```python
from build123d import *

# Parameters (mm, degrees)
SKETCH1_W           = 116.070000016
SKETCH1_H           = 84.320000016
BOSS_EXTRUDE1_DEPTH = 2.54
SKETCH2_W           = 116.070000016
SKETCH2_H           = 84.320000016
SKETCH2_W_2         = 108.450000016
SKETCH2_H_2         = 76.700000016
BOSS_EXTRUDE2_DEPTH = 34.925
CUT_EXTRUDE1_START  = 0.25
SKETCH4_R           = 1.349999967
CUT_EXTRUDE1_DEPTH  = 3.81
CUT_EXTRUDE2_START  = 0.25
SKETCH5_R           = 1.349999967
CUT_EXTRUDE2_DEPTH  = 3.81
SKETCH7_R           = 2.999999969
CUT_EXTRUDE3_DEPTH  = 2.000000064
SKETCH6_R           = 2.999999969
CUT_EXTRUDE4_DEPTH  = 2.000000064
CUT_EXTRUDE5_START  = 0.25
SKETCH11_W          = 22.225
SKETCH11_H          = 22.86
CUT_EXTRUDE5_DEPTH  = 3.81
CUT_EXTRUDE6_START  = 0.25
SKETCH8_W           = 22.225
SKETCH8_H           = 25.4
CUT_EXTRUDE6_DEPTH  = 3.81
CUT_EXTRUDE7_START  = 0.25
SKETCH10_W          = 22.225
SKETCH10_H          = 22.86
CUT_EXTRUDE7_DEPTH  = 3.81


with BuildPart() as part:
    # Sketch1 → Boss-Extrude1 (new body)
    with BuildSketch(Plane.YZ):
        Rectangle(SKETCH1_W, SKETCH1_H)
    extrude(amount=BOSS_EXTRUDE1_DEPTH)

    # Sketch2 → Boss-Extrude2 (add)
    with BuildSketch(Plane(origin=(0, 0, 0), x_dir=(0, -1, 0), z_dir=(-1, 0, 0))):
        Rectangle(SKETCH2_W, SKETCH2_H)
        Rectangle(SKETCH2_W_2, SKETCH2_H_2, mode=Mode.SUBTRACT)
    extrude(amount=BOSS_EXTRUDE2_DEPTH)

    # Sketch4 → Cut-Extrude1 (cut)
    with BuildSketch(Plane.XZ.offset(53.975).offset(CUT_EXTRUDE1_START)):
        with Locations((-28.575, 31.75)):
            Circle(SKETCH4_R)
        with Locations((-28.575, -31.75)):
            Circle(SKETCH4_R)
    extrude(amount=CUT_EXTRUDE1_DEPTH, mode=Mode.SUBTRACT)

    # Sketch5 → Cut-Extrude2 (cut)
    with BuildSketch(Plane(origin=(0, 53.975, 0), x_dir=(-1, 0, 0), z_dir=(0, 1, 0)).offset(CUT_EXTRUDE2_START)):
        with Locations((28.575, -31.75)):
            Circle(SKETCH5_R)
        with Locations((28.575, 31.75)):
            Circle(SKETCH5_R)
    extrude(amount=CUT_EXTRUDE2_DEPTH, mode=Mode.SUBTRACT)

    # Sketch7 → Cut-Extrude3 (cut)
    with BuildSketch(Plane(origin=(0, 58.035000008, 0), x_dir=(-1, 0, 0), z_dir=(0, 1, 0))):
        with Locations((28.575, -31.75)):
            Circle(SKETCH7_R)
        with Locations((28.575, 31.75)):
            Circle(SKETCH7_R)
    extrude(amount=-CUT_EXTRUDE3_DEPTH, mode=Mode.SUBTRACT)

    # Sketch6 → Cut-Extrude4 (cut)
    with BuildSketch(Plane.XZ.offset(58.035000008)):
        with Locations((-28.575, 31.75)):
            Circle(SKETCH6_R)
        with Locations((-28.575, -31.75)):
            Circle(SKETCH6_R)
    extrude(amount=-CUT_EXTRUDE4_DEPTH, mode=Mode.SUBTRACT)

    # Sketch11 → Cut-Extrude5 (cut)
    with BuildSketch(Plane(origin=(0, 0, -38.1), x_dir=(1, 0, 0), z_dir=(0, 0, -1)).offset(CUT_EXTRUDE5_START)):
        with Locations((-11.1125, 34.925)):
            Rectangle(SKETCH11_W, SKETCH11_H)
    extrude(amount=CUT_EXTRUDE5_DEPTH, mode=Mode.SUBTRACT)

    # Sketch8 → Cut-Extrude6 (cut)
    with BuildSketch(Plane.XZ.offset(53.975).offset(CUT_EXTRUDE6_START)):
        with Locations((-11.1125, -12.7)):
            Rectangle(SKETCH8_W, SKETCH8_H)
    extrude(amount=CUT_EXTRUDE6_DEPTH, mode=Mode.SUBTRACT)

    # Sketch10 → Cut-Extrude7 (cut)
    with BuildSketch(Plane.XY.offset(38.1).offset(CUT_EXTRUDE7_START)):
        with Locations((-11.1125, -34.925)):
            Rectangle(SKETCH10_W, SKETCH10_H)
    extrude(amount=CUT_EXTRUDE7_DEPTH, mode=Mode.SUBTRACT)


solid = part.part
```
Geometry check sheet. Reference: the model listing, model coordinates, mm. A direction names the side the tool comes from. Round coordinates to 2 decimals unless told otherwise and drop trailing zeros. Order: outer loops, then holes, each group sorted by start corner. A loop starts at its lowest first (then second) coordinate and runs counter-clockwise, first axis right, second up. Notation, with made-up numbers: M -26.75,-10.5 L 23.25,-10.5 A15 ccw 23.25,-2.5 Z; hole C 59,32.25 d5. An arc over 180 degrees is marked long. Answer as CSV lines item,"result".
1) Sectioned sample at C-C on z = 31.75. Record the cut outline in (x, y) (3 decimals).
Entries:
outline,"M -34.925,-58.035 L -31.575,-58.035 L -31.575,-56.035 L -29.925,-56.035 L -29.925,-54.225 L -34.925,-54.225 Z; M -34.925,54.225 L -29.925,54.225 L -29.925,56.035 L -31.575,56.035 L -31.575,58.035 L -34.925,58.035 Z; M -27.225,-56.035 L -25.575,-56.035 L -25.575,-58.035 L 2.54,-58.035 L 2.54,58.035 L -25.575,58.035 L -25.575,56.035 L -27.225,56.035 L -27.225,54.225 L 0,54.225 L 0,-54.225 L -27.225,-54.225 Z"
2) Sectioned sample at A-A on z = -18. Record the cut outline in (x, y) (3 decimals), and give its area (3 significant figures).
Entries:
outline,"M -34.925,-58.035 L -22.225,-58.035 L -22.225,-54.225 L -34.925,-54.225 Z; M -34.925,54.225 L 0,54.225 L 0,-58.035 L 2.54,-58.035 L 2.54,58.035 L -34.925,58.035 Z"
area,"476 mm2"
3) Sectioned sample at D-D on x = -12. Record the cut outline in (y, z) (3 decimals).
Entries:
outline,"M -58.035,-42.16 L -46.355,-42.16 L -46.355,-38.35 L -54.225,-38.35 L -54.225,-25.4 L -58.035,-25.4 Z; M -58.035,0 L -54.225,0 L -54.225,38.35 L -46.355,38.35 L -46.355,42.16 L -58.035,42.16 Z; M -23.495,-42.16 L 58.035,-42.16 L 58.035,42.16 L -23.495,42.16 L -23.495,38.35 L 54.225,38.35 L 54.225,-38.35 L -23.495,-38.35 Z"
4) Sectioned sample at B-B on y = -25.5. Record the cut outline in (x, z) (3 decimals).
Entries:
outline,"M -34.925,-42.16 L -22.225,-42.16 L -22.225,-38.35 L -34.925,-38.35 Z; M -34.925,38.35 L -22.225,38.35 L -22.225,42.16 L -34.925,42.16 Z; M 0,-42.16 L 2.54,-42.16 L 2.54,42.16 L 0,42.16 Z"
5) Tool access check on faces 4 (the face through (-17, 1, -38.35)), 5 (the face through (-11, -23.495, 40)), 6 (the face through (-25.804, -57.049, 30.601)). Record the directions out of +Z, -Z, +X, -X, +Y, -Y that give a thin tool (end or side, any length) a straight path to the whole face; none if there is none.
Entries:
face 4,"-X"
face 5,"+Z, -Z"
face 6,"-Y"
6) Gauge pin test, flat ends, axial feed: pin 1 Ø1.8 at (x, z) = (-27.5, -31.5) entering from +Y (3 decimals); pin 2 Ø1.8 at (x, z) = (-29, -32.5) entering from -Y (3 decimals); pin 3 Ø2.5 at (x, z) = (-28.575, 31.75) entering from -Y. Record the tip position at first contact, or that the pin passes through.
Entries:
pin 1,"y = 56.035"
pin 2,"y = -56.035"
pin 3,"through"
7) Thickness scan on probe 1 along Z at (x, y) = (-13.5, 48); probe 2 along Y at (x, z) = (-23, 8.5) (3 decimals); probe 3 along X at (y, z) = (-54.55, -31.75) (3 decimals). Record the ranges inside material, lowest first. Write a range as [from, to].
Entries:
probe 1,"[-42.16, -38.35], [38.35, 42.16]"
probe 2,"[-58.035, -54.225], [54.225, 58.035]"
probe 3,"[-34.925, -29.925], [-27.225, 2.54]"
8) Mould release check, pull along X, two halves, no side actions. Record for faces 1 (the face through (-22.225, -35, 40)), 2 (the face through (-17, -54.225, 8)), 3 (the face through (-11, -23.495, -40)): +X half, -X half, draft (parallel to the pull), parting line (faces both ways), or undercut.
Entries:
face 1,"undercut"
face 2,"draft"
face 3,"undercut"
